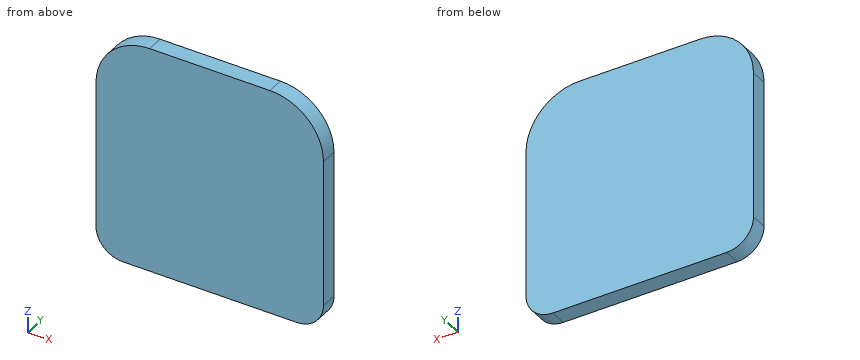
```python
from build123d import *

# Parameters (mm, degrees)
SKETCH1_W           = 85
SKETCH1_H           = 85
BOSS_EXTRUDE1_DEPTH = 6.3
FILLET1_R           = 10
FILLET2_R           = 20


with BuildPart() as part:
    # Sketch1 → Boss-Extrude1 (new body)
    with BuildSketch(Plane(origin=(0, 0, 0), x_dir=(1, 0, 0), z_dir=(0, 1, 0))):
        with Locations((42.5, 42.5)):
            Rectangle(SKETCH1_W, SKETCH1_H)
    extrude(amount=BOSS_EXTRUDE1_DEPTH)

    # Fillet1
    fillet1_edges = [part.edges().sort_by_distance(p)[0] for p in [
        (0, 3.15, -85),
        (85, 3.15, -85),
    ]]
    fillet(fillet1_edges, radius=FILLET1_R)

    # Fillet2
    fillet2_edges = [part.edges().sort_by_distance(p)[0] for p in [
        (85, 3.15, 0),
        (0, 3.15, 0),
    ]]
    fillet(fillet2_edges, radius=FILLET2_R)


solid = part.part
```
For this review, take the finished solid that the model builds, in its own axes (mm). Round coordinates to 2 decimals unless told otherwise and drop trailing zeros. Write each loop counter-clockwise with the first axis right and the second up, starting at its lowest first coordinate (ties: lowest second). Pieces come first, ordered by that corner, then holes. Notation, with made-up numbers: (-12, 72) - (24, 72) arc R24 ccw to (24, 104) - close; hole circle Ø4 at (13.5, 12.5). An arc over 180 degrees is marked (long way). Answer as a JSON object with one key per item and string values.
1. We need section C-C on x = 11. Give the boundary of the cut face in (y, z).
Response values:
{"outline": "(0, -85) - (6.3, -85) - (6.3, -2.14) - (0, -2.14) - close"}
2. To check wall thickness, follow line 1 along X through (y, z) = (0.75, -16.5); line 2 along X through (y, z) = (1, -15); line 3 along Z through (x, y) = (70.5, 1.5). State the ranges of each line that lie inside material, in increasing order.
Response values:
{"line 1": "x = 0.31 to 84.69", "line 2": "x = 0.64 to 84.36", "line 3": "z = -85 to -0.77"}
3. We need section A-A on y = 2. Give the boundary of the cut face in (x, z), then the cut area to 3 significant figures.
Response values:
{"outline": "(0, -75) arc R10 ccw to (10, -85) - (75, -85) arc R10 ccw to (85, -75) - (85, -20) arc R20 ccw to (65, 0) - (20, 0) arc R20 ccw to (0, -20) - close", "area": "7,010 mm2"}
4. We need section B-B on z = -14. Give the boundary of the cut face in (x, y), then the cut area to 3 significant figures.
Response values:
{"outline": "(0.92, 0) - (84.08, 0) - (84.08, 6.3) - (0.92, 6.3) - close", "area": "524 mm2"}
